Could you check a few things on this model? Use its own coordinates, in mm. Face numbers are marked on the shaded views. A direction names the side the tool comes from. Give positions to 0.01 mm unless a question says otherwise; leave off trailing zeros. Write each loop counter-clockwise with the first axis right and the second up, starting at its lowest first coordinate (ties: lowest second). Pieces come first, ordered by that corner, then holes. Notation, with made-up numbers: (67, -7.5) -> (76, -7.5) arc R26 cw to (76, 29.5) -> close; hole circle Ø10 at (-7.75, 60). An arc over 180 degrees is marked (long way). One line per question, with ' | ' between items.
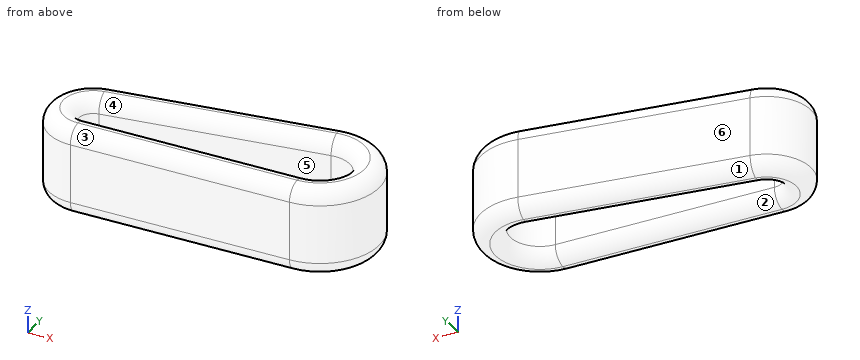
from build123d import *

# Parameters (mm, degrees)
F1_DEPTH = 30
F2_DEPTH = 25.4
F3_R     = 4.99999


# Not quite as in the source:
# - a fillet or chamfer is up to 0.001 mm smaller than in the source, because OpenCascade refuses the exact size


with BuildPart() as f1:
    # F0 (on Top) → F1 (new body)
    with BuildSketch(Plane.XY):
        with BuildLine():
            Line((34.7105600204, 69.6575524111), (-38.0615795526, 59.3297830847))
            ThreePointArc((-38.0615795526, 59.3297830847), (-50.9138983938, 43.3837240922), (-35.8768828371, 29.4787947456))
            Line((-35.8768828371, 29.4787947456), (37.6234889744, 29.8562346256))
            ThreePointArc((37.6234889744, 29.8562346256), (57.4674373389, 51.3158014327), (34.7105600204, 69.6575524111))
        make_face()
        with BuildLine():
            ThreePointArc((36.1156730696, 59.756761669), (47.4941117288, 50.5858861798), (37.5721375466, 39.8561027762))
            Line((37.5721375466, 39.8561027762), (-35.9282342649, 39.4786628962))
            ThreePointArc((-35.9282342649, 39.4786628962), (-40.9405727838, 44.1136393451), (-36.6564665034, 49.4289923426))
            Line((-36.6564665034, 49.4289923426), (36.1156730696, 59.756761669))
        make_face(mode=Mode.SUBTRACT)
    extrude(amount=F1_DEPTH)

    # F0 (on Top) → F2 (join)
    with BuildSketch(Plane.XY):
        with BuildLine():
            Line((34.7105600204, 69.6575524111), (-38.0615795526, 59.3297830847))
            ThreePointArc((-38.0615795526, 59.3297830847), (-50.9138983938, 43.3837240922), (-35.8768828371, 29.4787947456))
            Line((-35.8768828371, 29.4787947456), (37.6234889744, 29.8562346256))
            ThreePointArc((37.6234889744, 29.8562346256), (57.4674373389, 51.3158014327), (34.7105600204, 69.6575524111))
        make_face()
        with BuildLine():
            ThreePointArc((36.1156730696, 59.756761669), (47.4941117288, 50.5858861798), (37.5721375466, 39.8561027762))
            Line((37.5721375466, 39.8561027762), (-35.9282342649, 39.4786628962))
            ThreePointArc((-35.9282342649, 39.4786628962), (-40.9405727838, 44.1136393451), (-36.6564665034, 49.4289923426))
            Line((-36.6564665034, 49.4289923426), (36.1156730696, 59.756761669))
        make_face(mode=Mode.SUBTRACT)
    extrude(amount=F2_DEPTH)

    # F3 (radius 5 in the source; OpenCascade refuses exactly that, so slightly less here)
    f3_edges = [f1.edges().sort_by_distance(p)[0] for p in [
        (57.467437, 51.315801, 30),
        (-1.67551, 64.493668, 30),
        (-50.913898, 43.383724, 30),
        (0.873303, 29.667515, 30),
        (-40.940573, 44.113639, 30),
        (-0.270397, 54.592877, 30),
        (47.494112, 50.585886, 30),
        (0.821952, 39.667383, 30),
        (57.467437, 51.315801, 0),
        (-1.67551, 64.493668, 0),
        (-50.913898, 43.383724, 0),
        (0.873303, 29.667515, 0),
        (-40.940573, 44.113639, 0),
        (-0.270397, 54.592877, 0),
        (47.494112, 50.585886, 0),
        (0.821952, 39.667383, 0),
    ]]
    fillet(f3_edges, radius=F3_R)


solid = f1.part
Q1. If I drill on line 1 along Y through (x, z) = (-28.5, 14.75); line 2 along Y through (x, z) = (0.5, 28); line 3 along X through (y, z) = (43.5, 9.75), over which ranges is the centre line in solid material (lowest first)?
Answer below:
line 1: y = 29.52 to 39.52, 50.59 to 60.69 | line 2: y = 30.67 to 38.67, 55.71 to 63.79 | line 3: x = -50.92 to -40.86, 45.24 to 56.48
Q2. If we mould it in two halves opening along X, with no side actions, what happens to the marked faces 1 and 2? For each: +X half, -X half, draft (parallel to the pull), parting line (faces both ways), or undercut.
Answer below:
face 1: -X half | face 2: undercut
Q3. Will these pins go through, and if not, where does the flat tip stop? pin 1 (10 mm diameter, centred on x = -20, y = 43, fed in from -Z); pin 2 (10 mm diameter, centred on y = 35.5, z = 5, fed in from +X); pin 3 (8 mm diameter, centred on y = 62, z = 9, fed in from -X).
Answer below:
pin 1: stops at z = 1.37 | pin 2: stops at x = 55.2 | pin 3: stops at x = -42.45
Q4. On a 3-axis mill with a long thin cutter (end or side, diameter ignored), from which of +Z, -Z, +X, -X, +Y, -Y can I reach the whole of each face in a straight line? I mean the marked faces 3, 4, 5 and 6. Say none if no direction works.
Answer below:
face 3: +Z, +X, -Y | face 4: +Z | face 5: +Z, -Z | face 6: +Z, -Z, -X, +Y
Q5. Imagine slicing it at A-A on z = 7. Please give me the cut outline in (x, y), and give its area (3 significant figures).
Answer below:
outline: (-38.06, 59.33) arc R15 ccw to (-35.88, 29.48) -> (37.62, 29.86) arc R20 ccw (long way) to (34.71, 69.66) -> close; hole (-36.66, 49.43) arc R5 ccw to (-35.93, 39.48) -> (37.57, 39.86) arc R10 ccw (long way) to (36.12, 59.76) -> close | area: 2,260 mm^2
